The listing builds one solid part. Answer for the finished solid, in the listing's coordinates (mm). Face numbers are marked on the shaded views. A direction names the side the tool comes from. Coordinates: 2 decimals unless noted, no trailing zeros. Write each loop counter-clockwise with the first axis right and the second up, starting at its lowest first coordinate (ties: lowest second). Pieces come first, ordered by that corner, then holes. Notation, with made-up numbers: M 65,10.25 L 97,10.25 A15 ccw 97,22.25 Z; hole C -0.75,40.25 d5. An arc over 180 degrees is marked long. Answer as CSV lines item,"result".
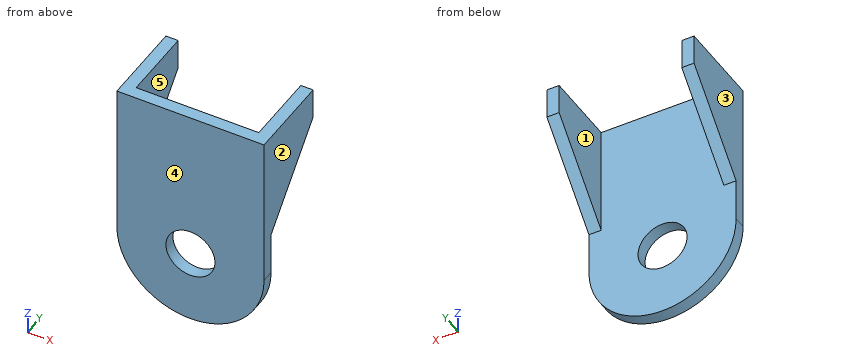
```python
from build123d import *

# Parameters (mm, degrees)
SKETCH_1_R      = 12
SKETCH_1_R_2    = 4
EXTRUDE_1_DEPTH = 2
EXTRUDE_2_DEPTH = 2


with BuildPart() as part:
    # 草图1 → 凸台-拉伸1 (new body)
    # profile 1 of 2: a face of its own
    with BuildSketch(Plane(origin=(0, 0, 0), x_dir=(1, 0, 0), z_dir=(0, 1, 0))):
        Circle(SKETCH_1_R)
        with Locations(Location((0, 0, 0), (0, 0, 270))):
            Circle(SKETCH_1_R_2, mode=Mode.SUBTRACT)
    # profile 2 of 2: a face of its own
    with BuildSketch(Plane(origin=(0, 0, 0), x_dir=(1, 0, 0), z_dir=(0, 1, 0))):
        with BuildLine():
            ThreePointArc((12, 0), (0, -12), (-12, 0))
            Line((-12, 0), (-12, -25))
            Line((-12, -25), (12, -25))
            Line((12, -25), (12, 0))
        make_face()
    extrude(amount=EXTRUDE_1_DEPTH)

    # 草图3 → 凸台-拉伸2 (add)
    with BuildSketch(Plane(origin=(12, 0, 0), x_dir=(0, 0, -1), z_dir=(1, 0, 0))):
        Polygon((-25, 2), (-25, 14), (-20, 14), (-7, 2), align=None)
    extrude_2 = extrude(amount=-EXTRUDE_2_DEPTH)

    # 镜向1: 凸台-拉伸2 across plane
    add(extrude_2.mirror(Plane(origin=(0, 0, 0), x_dir=(0, 0, 1), z_dir=(1, 0, 0))))


solid = part.part
```
Q1. Straight lines are drawn through the part: line 1 (X direction, y = 0.75, z = 0); line 2 (Y direction, x = 1, z = -4); line 3 (Z direction, x = -6, y = 1). For each, find the intervals that lie inside material, in ascending order.
Output:
line 1,"-12 to -4, 4 to 12"
line 2,"0 to 2"
line 3,"-10.39 to 25"
Q2. For the marked faces 1 and 2, determine the directions among +Z, -Z, +X, -X, +Y, -Y from which every point of the face is accessible in a straight line to the end or side of a thin tool.
Output:
face 1,"+Z, -Z, +Y"
face 2,"+Z, -Z, +X, +Y, -Y"
Q3. Find section C-C (z = 23). Give the vertices of the cut face in (x, y), and give its area (3 significant figures).
Output:
outline,"M -12,0 L 12,0 L 12,14 L 10,14 L 10,2 L -10,2 L -10,14 L -12,14 Z"
area,"96.0 mm2"
Q4. Flat-ended cylindrical pins translate along their axes: pin 1 Ø5 at (x, z) = (4.5, -2) entering from +Y; pin 2 Ø5 at (x, z) = (0, 0) entering from -Y. Find the tip coordinate at first contact, or state that the pin passes through.
Output:
pin 1,"y = 2"
pin 2,"through"
Q5. Find section B-B (y = 9.5). Give the vertices of the cut face in (x, z) (3 decimals), and give its area (3 significant figures).
Output:
outline,"M -12,15.125 L -10,15.125 L -10,25 L -12,25 Z; M 10,15.125 L 12,15.125 L 12,25 L 10,25 Z"
area,"39.5 mm2"
Q6. Find section A-A (x = 0). Give the vertices of the cut face in (y, z), and give its area (3 significant figures).
Output:
outline,"M 0,-12 L 2,-12 L 2,-4 L 0,-4 Z; M 0,4 L 2,4 L 2,25 L 0,25 Z"
area,"58.0 mm2"
Q7. The mould has two halves that part along X. Classify the marked faces 3, 4 and 5: pulls with the +X half, pulls with the -X half, needs draft (parallel to the pull), parting line crosses it, or undercut.
Output:
face 3,"pulls with the -X half"
face 4,"needs draft"
face 5,"undercut"
Q8. Find section D-D (z = 14). Give the vertices of the cut face in (x, y).
Output:
outline,"M -12,0 L 12,0 L 12,8.46 L 10,8.46 L 10,2 L -10,2 L -10,8.46 L -12,8.46 Z"
